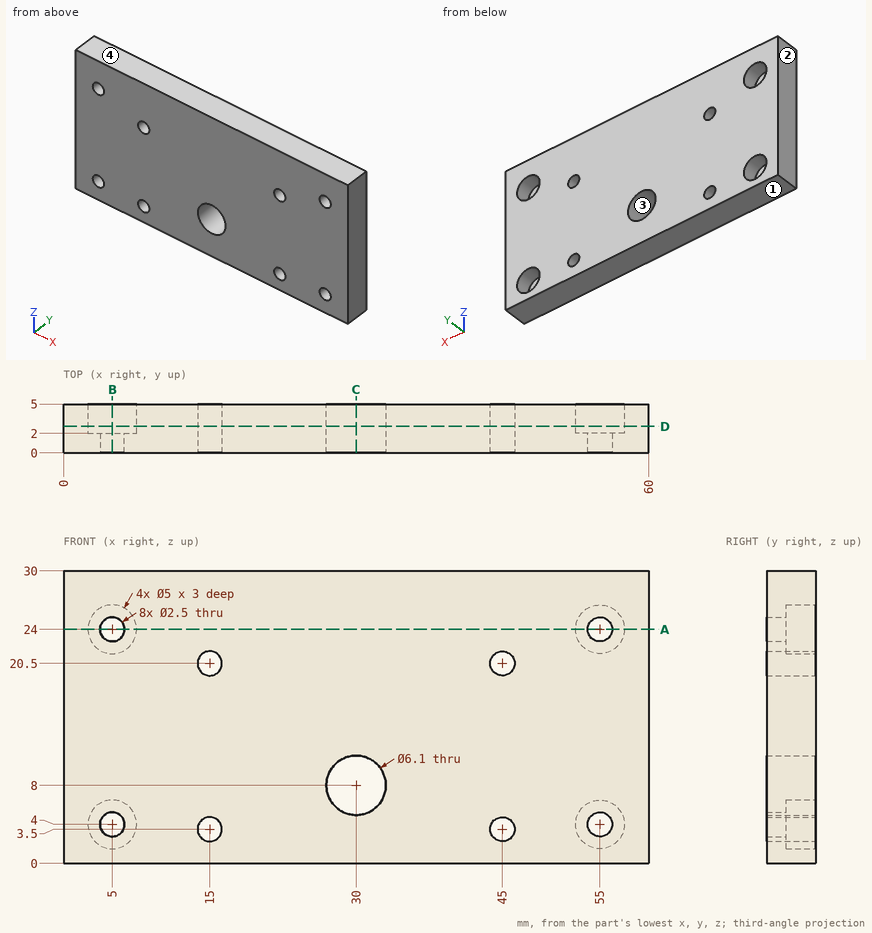
Drawing for the job (mm, zero at the part's lowest x, y, z). Round coordinates to 2 decimals unless told otherwise and drop trailing zeros. Write each loop counter-clockwise with the first axis right and the second up, starting at its lowest first coordinate (ties: lowest second). Pieces come first, ordered by that corner, then holes. Notation, with made-up numbers: M -11.5,75.5 L 27.5,75.5 A33 cw 27.5,112.5 Z; hole C 88,-12.75 d8. An arc over 180 degrees is marked long. Answer as a JSON object with one key per item and string values. Group by question number.
(1) Flat gauge pins, fed straight in: pin 1 (4 mm diameter, centred on x = 45, z = 3.5, fed in from +Y); pin 2 (3 mm diameter, centred on x = 5, z = 4, fed in from +Y). Where does each tip first touch, or does it go through?
(2) Cut at D-D (y = 2.7). Give the number of separate pieces and of enclosed holes in the cut face, and give its area (3 significant figures).
(3) Drill centre lines: L1, parallel to Z at x = 15, y = 2.5; L2, parallel to Z at x = 5, y = 1.35; L3, parallel to X at y = 1.15, z = 20.5. Where is each one in solid material? Low to high.
(4) Mould opens along Z. For the marked faces 1, 2, 3 and 4 say: pulls with the +Z half, pulls with the -Z half, needs draft (parallel to the pull), parting line crosses it, or undercut.
(5) Cut at C-C (x = 30). Give the cut face in (y, z), and give its area (4 significant figures).
(6) Cut at A-A (z = 24). Give the cut face in (x, y), and give its area (3 significant figures).
(7) Cut at B-B (x = 5). Give the cut face in (y, z).
Responses:
{
 "1": {"pin 1": "stops at y = 5", "pin 2": "stops at y = 2"},
 "2": {"separate pieces": "1", "enclosed holes": "9", "area": "1,670 mm2"},
 "3": {"L1": "z = 0 to 2.25, 4.75 to 19.25, 21.75 to 30", "L2": "z = 0 to 2.75, 5.25 to 22.75, 25.25 to 30", "L3": "x = 0 to 13.75, 16.25 to 43.75, 46.25 to 60"},
 "4": {"face 1": "pulls with the -Z half", "face 2": "needs draft", "face 3": "undercut", "face 4": "pulls with the +Z half"},
 "5": {"outline": "M 0,0 L 5,0 L 5,4.95 L 0,4.95 Z; M 0,11.05 L 5,11.05 L 5,30 L 0,30 Z", "area": "119.5 mm2"},
 "6": {"outline": "M 0,0 L 3.75,0 L 3.75,2 L 2.5,2 L 2.5,5 L 0,5 Z; M 6.25,0 L 53.75,0 L 53.75,2 L 52.5,2 L 52.5,5 L 7.5,5 L 7.5,2 L 6.25,2 Z; M 56.25,0 L 60,0 L 60,5 L 57.5,5 L 57.5,2 L 56.25,2 Z", "area": "260 mm2"},
 "7": {"outline": "M 0,0 L 5,0 L 5,1.5 L 2,1.5 L 2,2.75 L 0,2.75 Z; M 0,5.25 L 2,5.25 L 2,6.5 L 5,6.5 L 5,21.5 L 2,21.5 L 2,22.75 L 0,22.75 Z; M 0,25.25 L 2,25.25 L 2,26.5 L 5,26.5 L 5,30 L 0,30 Z"}
}
